The drawing under review shows one solid part. Ordinate dimensions are in mm from its lowest x, y, z. A direction names the side the tool comes from. Give positions to 0.01 mm unless a question says otherwise; leave off trailing zeros. Write each loop counter-clockwise with the first axis right and the second up, starting at its lowest first coordinate (ties: lowest second). Pieces come first, ordered by that corner, then holes.
Q1. We need section A-A (x = 40). Write out the cut boundary in (y, z), then the cut area to 3 significant figures.
Q2. For line 1 (Z direction, x = 38, y = 107); line 2 (X direction, y = 54, z = 38) (1 decimal); line 3 (X direction, y = 64, z = 43) (1 decimal), list the stretches that pass through material, from the lowest coordinate up.
Q3. Insertion check: P1, Ø10, axis at y = 49, z = 41, coming from the +X side; P2, Ø4, axis at x = 36, z = 42, coming from the +Y side. Each pin has a flat end and moves straight along its axis. Give the tip position at first contact, or say it passes through.
Q4. We need section C-C (z = 47). Write out the cut boundary in (x, y) (1 decimal), then the cut area to 3 significant figures.
Q5. Machinability: for the marked faces 1 and 2, which of the approach directions +Z, -Z, +X, -X, +Y, -Y give a long, thin tool a straight path to every point of the face, cutting with its end or side? Answer none if there is none.
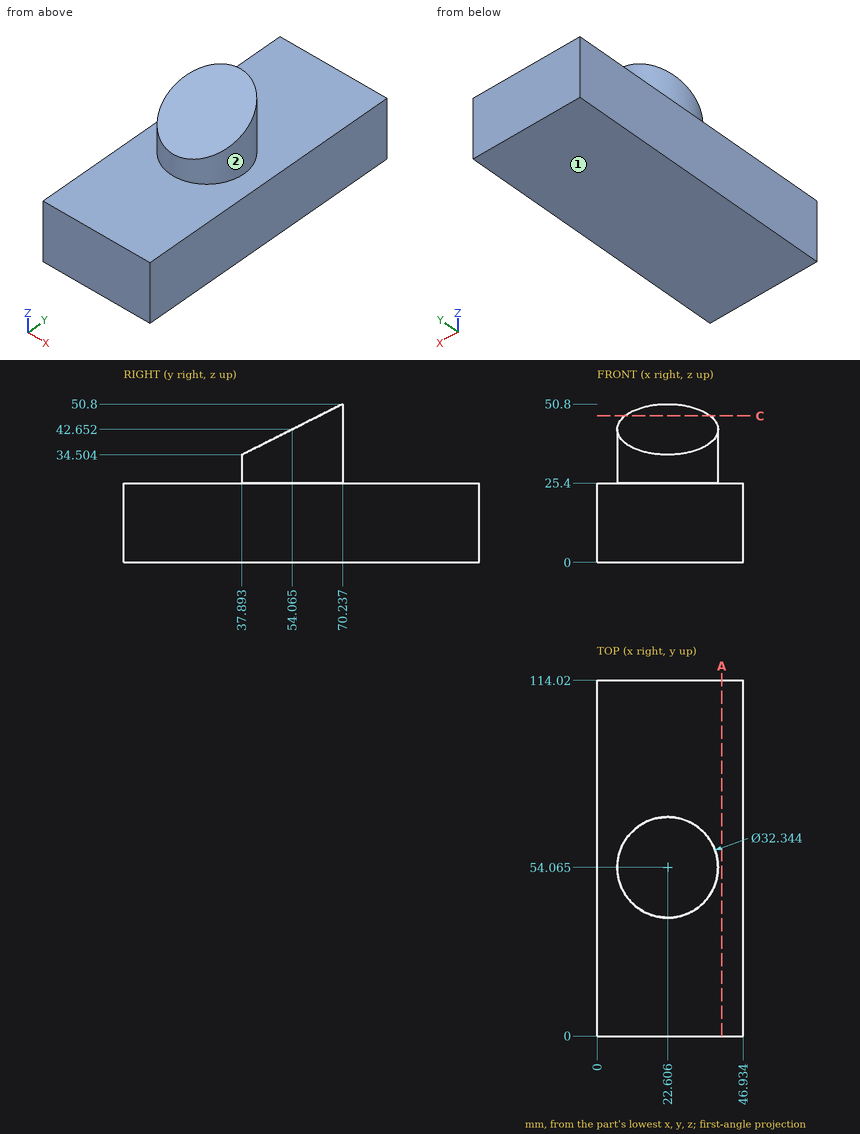
Computed:
1. outline: (0, 0) - (114.02, 0) - (114.02, 25.4) - (0, 25.4) - close
1. area: 2,900 mm2
2. line 1: z = 0 to 25.4
2. line 2: x = 6.4 to 38.8
2. line 3: x = 9.8 to 35.4
3. P1: stops at x = 38.78
3. P2: stops at y = 65.54
4. outline: (8.9, 62.7) - (36.3, 62.7) arc R16.2 ccw to start
4. area: 146 mm2
5. face 1: -Z, +X, -X, +Y, -Y
5. face 2: +Z
